Geometry check sheet. Reference: the model listing, model coordinates, mm. Face numbers are marked on the shaded views. Coordinates: 2 decimals unless noted, no trailing zeros. Write each loop counter-clockwise with the first axis right and the second up, starting at its lowest first coordinate (ties: lowest second). Pieces come first, ordered by that corner, then holes. Notation, with made-up numbers: (2, 14.25) -> (39, 14.25) arc R26 ccw to (39, 39.25) -> close; hole circle Ø8 at (10.5, 47.25). An arc over 180 degrees is marked (long way). Answer in a Markdown table with one row per item. Add a question column.
1. Mould release check, pull along Y, two halves, no side actions. Record for the marked faces 1, 2 and 3: pulls with the +Y half, pulls with the -Y half, needs draft (parallel to the pull), parting line crosses it, or undercut.
2. Scan lines: L1, parallel to Y at x = 2, z = 3; L2, parallel to Y at x = -14.55, z = -10; L3, parallel to X at y = 9.25, z = -10.25. Record each from-to range of solid material in increasing order. Write a range as from..to.
3. Cross-section at B-B on x = 17. Record the cut outline in (y, z), and give its area (3 significant figures).
4. Cross-section at C-C on y = 3.25. Record the cut outline in (x, z).
5. Cross-section at A-A on z = 2. Record the cut outline in (x, y), and give its area (3 significant figures).
6. Cross-section at D-D on x = -5. Record the cut outline in (y, z), and give its area (3 significant figures).
7. Depth check by flat-ended pin: P1, Ø5, axis at y = 7, z = -5.5, coming from the +X side; P2, Ø1.1, axis at y = -0.5, z = -4, coming from the -X side; P3, Ø1, axis at x = 14, z = -8.5, coming from the +Y side; P4, Ø2.5, axis at y = 5.53, z = -10, coming from the +X side. Enter the tip coordinate at first touch or a pass-through.
```python
from build123d import *

# Parameters (mm, degrees)
SKETCH_1_R             = 1.5
SM_BASE_FLANGE_1_DEPTH = 1
OTHER_START            = -25
OTHER_1_OUTLINE_W      = 1
OTHER_1_OUTLINE_H      = 30
OTHER_1_DEPTH          = 10
OTHER_START_2          = -14.831098284
OTHER_1_2_OUTLINE_R    = 1.5
OTHER_1_2_DEPTH        = 0.831098284
OTHER_START_3          = -15
OTHER_1_3_OUTLINE_R    = 1.5
OTHER_1_3_DEPTH        = 1.7366
OTHER_1_4_DEPTH        = 30


with BuildPart() as part:
    # 基体-法兰1: sheet metal written as solids
    # Sketch 1 → 基体-法兰1 (new body)
    with BuildSketch(Plane(origin=(0, 0, 0), x_dir=(1, 0, 0), z_dir=(0, 1, 0))):
        with BuildLine():
            Line((-24, 15), (24, 15))
            ThreePointArc((24, 15), (24.707106781, 14.707106781), (25, 14))
            Line((25, 14), (25, -14))
            ThreePointArc((25, -14), (24.707106781, -14.707106781), (24, -15))
            Line((24, -15), (-24, -15))
            ThreePointArc((-24, -15), (-24.707106781, -14.707106781), (-25, -14))
            Line((-25, -14), (-25, 14))
            ThreePointArc((-25, 14), (-24.707106781, 14.707106781), (-24, 15))
        make_face()
        with Locations(Location((-20, -10, 0), (0, 0, 270))):
            Circle(SKETCH_1_R, mode=Mode.SUBTRACT)
        with Locations(Location((-20, 10, 0), (0, 0, 270))):
            Circle(SKETCH_1_R, mode=Mode.SUBTRACT)
        with BuildLine():
            Line((-3.5, -10), (-3.5, 10))
            ThreePointArc((-3.5, 10), (-2, 11.5), (-0.5, 10))
            Line((-0.5, 10), (-0.5, -10))
            ThreePointArc((-0.5, -10), (-2, -11.5), (-3.5, -10))
        make_face(mode=Mode.SUBTRACT)
        with BuildLine():
            Line((15.5, -10), (15.5, 10))
            ThreePointArc((15.5, 10), (17, 11.5), (18.5, 10))
            Line((18.5, 10), (18.5, -10))
            ThreePointArc((18.5, -10), (17, -11.5), (15.5, -10))
        make_face(mode=Mode.SUBTRACT)
    extrude(amount=-SM_BASE_FLANGE_1_DEPTH)

    # Other 1: read off the stored shape, not the designer's step
    # Other 1 outline → Other 1 (cut)
    with BuildSketch(Plane.YZ.offset(OTHER_START)):
        with Locations((-0.5, 0)):
            Rectangle(OTHER_1_OUTLINE_W, OTHER_1_OUTLINE_H)
    extrude(amount=OTHER_1_DEPTH, mode=Mode.SUBTRACT)

    # Other 1 2 outline → Other 1 2 (add)
    with BuildSketch(Plane.YZ.offset(OTHER_START_2)):
        with BuildLine():
            ThreePointArc((10.530753262, 14), (10.237860043, 14.707106781), (9.530753262, 15))
            Line((9.530753262, 15), (0, 15))
            Line((0, 15), (0, -15))
            Line((0, -15), (9.530753262, -15))
            ThreePointArc((9.530753262, -15), (10.237860043, -14.707106781), (10.530753262, -14))
            Line((10.530753262, -14), (10.530753262, 14))
        make_face()
        with Locations((5.530753262, -10)):
            Circle(OTHER_1_2_OUTLINE_R, mode=Mode.SUBTRACT)
        with Locations((5.530753262, 10)):
            Circle(OTHER_1_2_OUTLINE_R, mode=Mode.SUBTRACT)
    extrude(amount=OTHER_1_2_DEPTH)

    # Other 1 3 outline → Other 1 3 (add)
    with BuildSketch(Plane.YZ.offset(OTHER_START_3)):
        with BuildLine():
            ThreePointArc((10.530753262, 14), (10.237860043, 14.707106781), (9.530753262, 15))
            Line((9.530753262, 15), (0, 15))
            Line((0, 15), (0, -15))
            Line((0, -15), (9.530753262, -15))
            ThreePointArc((9.530753262, -15), (10.237860043, -14.707106781), (10.530753262, -14))
            Line((10.530753262, -14), (10.530753262, 14))
        make_face()
        with Locations((5.530753262, -10)):
            Circle(OTHER_1_3_OUTLINE_R, mode=Mode.SUBTRACT)
        with Locations((5.530753262, 10)):
            Circle(OTHER_1_3_OUTLINE_R, mode=Mode.SUBTRACT)
    extrude(amount=OTHER_1_3_DEPTH)

    # Other 1 4 outline → Other 1 4 (cut)
    with BuildSketch(Plane.XY.offset(OTHER_START_3)):
        with BuildLine():
            ThreePointArc((-13.2634, -1), (-14.491361636, -0.491361636), (-15, 0.7366))
            Line((-15, 0.7366), (-15, -1))
            Line((-15, -1), (-13.2634, -1))
        make_face()
        with BuildLine():
            Line((-14, 10.530753262), (-14, 0.7366))
            ThreePointArc((-14, 0.7366), (-13.784254855, 0.215745145), (-13.2634, 0))
            Line((-13.2634, 0), (-13.2634, 10.530753262))
            Line((-13.2634, 10.530753262), (-14, 10.530753262))
        make_face()
    extrude(amount=OTHER_1_4_DEPTH, mode=Mode.SUBTRACT)


solid = part.part
```
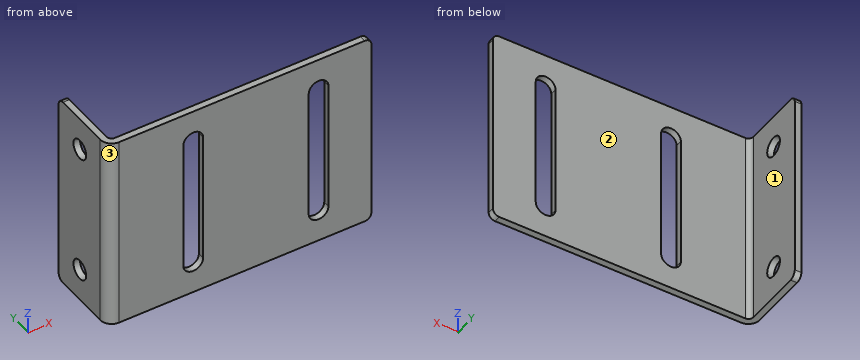
Results found:
| question | item | result |
|---|---|---|
| 1 | face 1 | needs draft |
| 1 | face 2 | pulls with the +Y half |
| 1 | face 3 | pulls with the -Y half |
| 2 | L1 | y = -1..0 |
| 2 | L2 | y = -0.43..4.03, 7.03..10.53 |
| 2 | L3 | x = -15..-14 |
| 3 | outline | (-1, -15) -> (0, -15) -> (0, -11.5) -> (-1, -11.5) -> close; (-1, 11.5) -> (0, 11.5) -> (0, 15) -> (-1, 15) -> close |
| 3 | area | 7.00 mm^2 |
| 4 | outline | (-15, -15) -> (-14, -15) -> (-14, 15) -> (-15, 15) -> close |
| 5 | outline | (-15, 0.74) arc R1.74 ccw to (-13.26, -1) -> (-3.5, -1) -> (-3.5, 0) -> (-13.26, 0) arc R0.74 cw to (-14, 0.74) -> (-14, 10.53) -> (-15, 10.53) -> close; (-0.5, -1) -> (15.5, -1) -> (15.5, 0) -> (-0.5, 0) -> close; (18.5, -1) -> (25, -1) -> (25, 0) -> (18.5, 0) -> close |
| 5 | area | 44.0 mm^2 |
| 6 | outline | (-1, -15) -> (0, -15) -> (0, 15) -> (-1, 15) -> close |
| 6 | area | 30.0 mm^2 |
| 7 | P1 | stops at x = -14 |
| 7 | P2 | stops at x = -14.86 |
| 7 | P3 | stops at y = 0 |
| 7 | P4 | passes through |
